Could you check a few things on this model? Use its own coordinates, in mm. A direction names the side the tool comes from. Give positions to 0.01 mm unless a question says otherwise; leave off trailing zeros. Write each loop counter-clockwise with the first axis right and the second up, starting at its lowest first coordinate (ties: lowest second). Pieces come first, ordered by that corner, then holes. Notation, with made-up numbers: (43.25, 46) - (50.25, 46) arc R25 cw to (50.25, 85) - close; hole circle Ø9 at (74, 13). An arc over 180 degrees is marked (long way). Answer in a Markdown table with one row per item.
from build123d import *

# Parameters (mm, degrees)
F1_W     = 152.4
F1_H     = 76.2
F2_DEPTH = 76.2
F3_W     = 76.2
F3_H     = 76.2
F4_DEPTH = 76.2
F5_W     = 76.2
F5_H     = 76.2
F6_DEPTH = 76.2


# Not quite as in the source:
# - a variable given as a bare number and used for a length is read in inches; the dataset says mm whatever the document's units were


with BuildPart() as f2:
    # F1 (on Front) → F2 (new body)
    with BuildSketch(Plane.XZ):
        with Locations((0, -5.0575301152)):
            Rectangle(F1_W, F1_H)
    extrude(amount=F2_DEPTH)

    # F3 (on face) → F4 (join)
    with BuildSketch(Plane(origin=(0, 0, 0), x_dir=(-1, 0, 0), z_dir=(0, 1, 0))):
        with Locations((38.1, -5.0575301152)):
            Rectangle(F3_W, F3_H)
    extrude(amount=F4_DEPTH)

    # F5 (on face) → F6 (join)
    with BuildSketch(Plane.XY.offset(33.0424698848)):
        with Locations((-38.1, 38.1)):
            Rectangle(F5_W, F5_H)
    extrude(amount=F6_DEPTH)


solid = f2.part
1) Will these pins go through, and if not, where does the flat tip stop? P1, Ø2, axis at x = 43.5, y = -11.5, coming from the +Z side; P2, Ø23, axis at x = -47, z = 52.5, coming from the -Y side.
Check values:
| item | result |
|---|---|
| P1 | stops at z = 33.04 |
| P2 | stops at y = 0 |
2) Imagine slicing it at A-A (z = -24.5). List the corners of the cut face in (x, y) for me.
Check values:
| item | result |
|---|---|
| outline | (-76.2, -76.2) - (76.2, -76.2) - (76.2, 0) - (0, 0) - (0, 76.2) - (-76.2, 76.2) - close |
3) Imagine slicing it at D-D (z = 62.5). List the corners of the cut face in (x, y) for me.
Check values:
| item | result |
|---|---|
| outline | (-76.2, 0) - (0, 0) - (0, 76.2) - (-76.2, 76.2) - close |
4) If I drill on line 1 (Y direction, x = -35.5, z = 39); line 2 (Z direction, x = 38.5, y = -0.5); line 3 (Y direction, x = 68.5, z = -1), over which ranges is the centre line in solid material (lowest first)?
Check values:
| item | result |
|---|---|
| line 1 | y = 0 to 76.2 |
| line 2 | z = -43.16 to 33.04 |
| line 3 | y = -76.2 to 0 |
5) On a 3-axis mill with a long thin cutter (end or side, diameter ignored), from which of +Z, -Z, +X, -X, +Y, -Y can I reach the whole of each face in a straight line? I mean faces 1 (the face through (-76.2, 16, 15)), 2 (the face through (1, -39, 33.042)), 3 (the face through (0, 38, 32)). Say none if no direction works.
Check values:
| item | result |
|---|---|
| face 1 | +Z, -Z, -X, +Y, -Y |
| face 2 | +Z, +X, -X, -Y |
| face 3 | +Z, -Z, +X, +Y |
6) Imagine slicing it at C-C (y = -52). List the corners of the cut face in (x, z) for me.
Check values:
| item | result |
|---|---|
| outline | (-76.2, -43.16) - (76.2, -43.16) - (76.2, 33.04) - (-76.2, 33.04) - close |
7) Imagine slicing it at B-B (x = -17). List the corners of the cut face in (y, z) for me, then the cut area to 3 significant figures.
Check values:
| item | result |
|---|---|
| outline | (-76.2, -43.16) - (76.2, -43.16) - (76.2, 109.24) - (0, 109.24) - (0, 33.04) - (-76.2, 33.04) - close |
| area | 17,400 mm2 |
